The model under review builds one solid part; all positions refer to its coordinate system, in mm. Coordinates: 2 decimals unless noted, no trailing zeros. Write each loop counter-clockwise with the first axis right and the second up, starting at its lowest first coordinate (ties: lowest second). Pieces come first, ordered by that corner, then holes. Notation, with made-up numbers: (76, 37.25) - (81, 37.25) arc R24 cw to (81, 54.25) - close; hole circle Ø7 at (81, 80). An arc over 180 degrees is marked (long way). Put each result on its own line as item: value. Start each with the question number.
Item 1: Consider section A-A on z = 1.25. State how many separate pieces and enclosed holes the cut face has, then the cut area to 3 significant figures.
Item 2: To check wall thickness, follow L1, parallel to Y at x = -15.5, z = 2; L2, parallel to X at y = -39, z = 2; L3, parallel to X at y = 4.5, z = 1.5. State the ranges of each line that lie inside material, in increasing order. Write a range as [from, to].
Item 3: Consider section B-B on y = -44.5. Give the boundary of the cut face in (x, z) (3 decimals), then the cut area to 3 significant figures.
Item 4: For pin 1 (1 mm diameter, centred on x = -59, z = 1.5, fed in from +Y); pin 2 (1 mm diameter, centred on x = -6, z = 0.5, fed in from +Y), all flat-tipped, find the tip position at first contact; note any pin that passes through.
Item 5: Consider section C-C on x = 41. Give the boundary of the cut face in (y, z) (3 decimals).
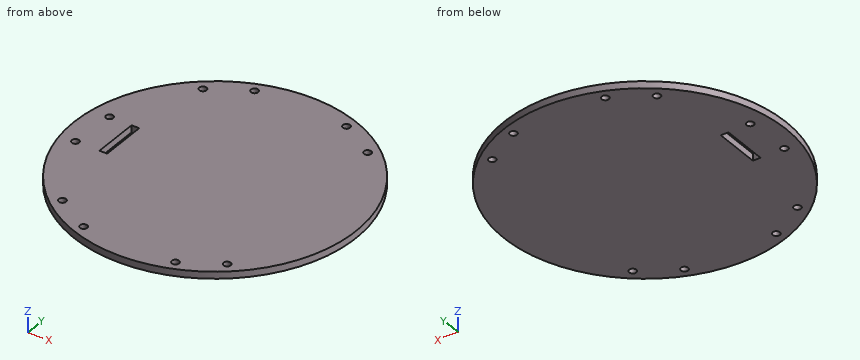
```python
from build123d import *

# Parameters (mm, degrees)
SKETCH1_R           = 64.5
SKETCH1_R_2         = 1.65
SKETCH1_W           = 3.5
SKETCH1_H           = 21
BOSS_EXTRUDE1_DEPTH = 3.175


with BuildPart() as part:
    # Sketch1 → Boss-Extrude1 (new body)
    with BuildSketch(Plane(origin=(0, 0, 0), x_dir=(-1, 0, 0), z_dir=(0, 0, 1))):
        with Locations((14.94226781, -5.633574242)):
            Circle(SKETCH1_R)
        with Locations((-6.05773219, 50.366425758)):
            Circle(SKETCH1_R_2, mode=Mode.SUBTRACT)
        with Locations((-22.69188657, 40.366425758)):
            Circle(SKETCH1_R_2, mode=Mode.SUBTRACT)
        with Locations((35.94226781, 50.366425758)):
            Circle(SKETCH1_R_2, mode=Mode.SUBTRACT)
        with Locations((52.57642219, 40.366425758)):
            Circle(SKETCH1_R_2, mode=Mode.SUBTRACT)
        with Locations((52.57642219, -51.633574242)):
            Circle(SKETCH1_R_2, mode=Mode.SUBTRACT)
        with Locations((35.94226781, -61.633574242)):
            Circle(SKETCH1_R_2, mode=Mode.SUBTRACT)
        with Locations((-6.05773219, -61.633574242)):
            Circle(SKETCH1_R_2, mode=Mode.SUBTRACT)
        with Locations((-22.69188657, -51.633574242)):
            Circle(SKETCH1_R_2, mode=Mode.SUBTRACT)
        with Locations((71.403979127, 4.866425758)):
            Circle(SKETCH1_R_2, mode=Mode.SUBTRACT)
        with Locations((70.44226781, -16.133574242)):
            Circle(SKETCH1_R_2, mode=Mode.SUBTRACT)
        with Locations((58.69226781, -5.633574242)):
            Rectangle(SKETCH1_W, SKETCH1_H, mode=Mode.SUBTRACT)
    extrude(amount=BOSS_EXTRUDE1_DEPTH)


solid = part.part
```
Report:
1. separate pieces: 1
1. enclosed holes: 11
1. area: 12,900 mm²
2. L1: [-58.86, 70.13]
2. L2: [-61.51, -53.5], [-51.65, 21.77], [23.62, 31.62]
2. L3: [-79.43, -60.44], [-56.94, 49.55]
3. outline: (-55.524, 0) - (25.639, 0) - (25.639, 3.175) - (-55.524, 3.175) - close
3. area: 258 mm²
4. pin 1: y = 53.2
4. pin 2: y = 69.58
5. outline: (-26.471, 0) - (37.738, 0) - (37.738, 3.175) - (-26.471, 3.175) - close
